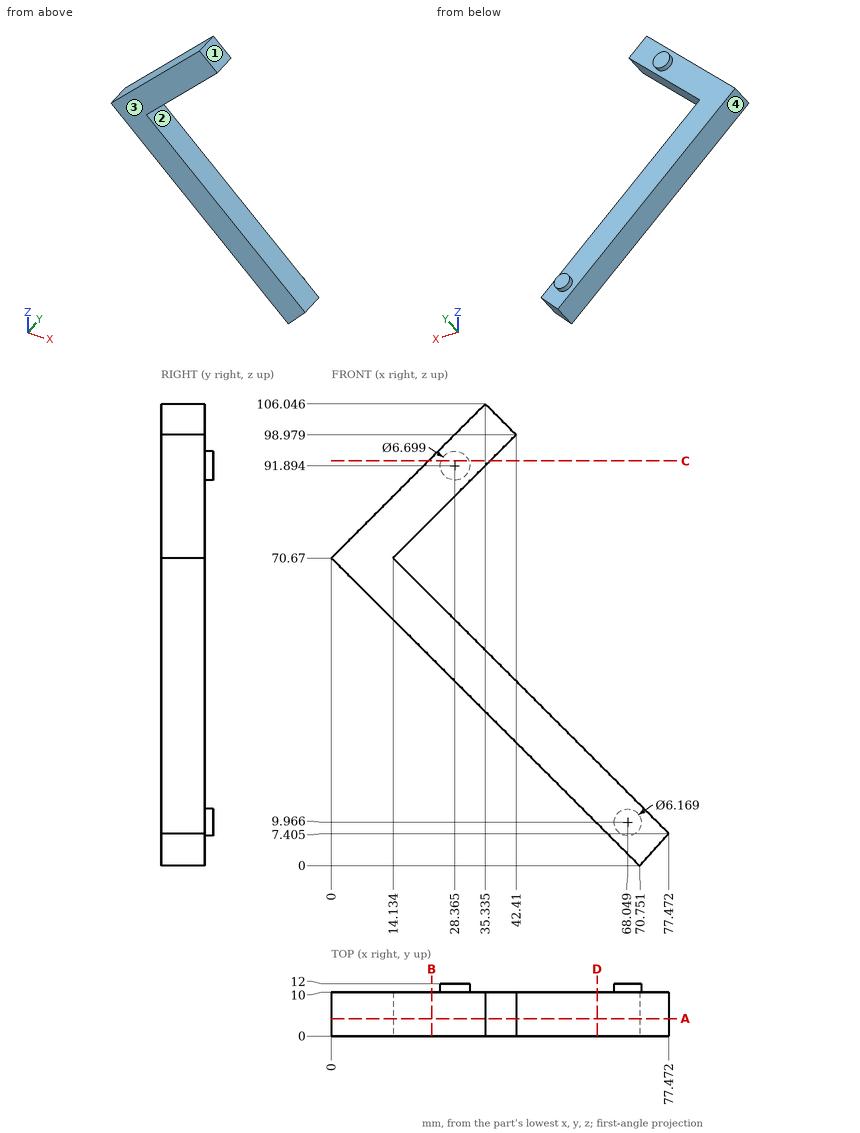
Source: three-view drawing plus pictorial views. Frame: mm from the lowest corner of the part. Coordinates: 2 decimals unless noted, no trailing zeros. Loops run counter-clockwise (first coordinate to the right, second up) from the corner with the lowest first, then second, coordinate; pieces in that order, holes last. Notation, with made-up numbers: (75.25, -22.5) - (108.25, -22.5) arc R28 ccw to (108.25, -1.5) - close; hole circle Ø3 at (-20, -22.75). An arc over 180 degrees is marked (long way). Answer in a Markdown table with one row per item. Add a question column.
Item 1: Section query C-C on z = 93. Return the cut outline in (x, y) (1 decimal), then the cut area to 3 significant figures.
Item 2: Line query: line 1 along Z through (x, y) = (37.5, 6.75) (1 decimal); line 2 along Z through (x, y) = (31.5, 6) (1 decimal); line 3 along Y through (x, z) = (36, 38.5). Output: solid intervals per line, ascending. Write a range as [from, to].
Item 3: Section query A-A on y = 4. Return the cut outline in (x, z) (1 decimal).
Item 4: Section query B-B on x = 23. Return the cut outline in (y, z) (1 decimal).
Item 5: Contact query for flat-ended pins moving along their axis: P1, Ø4, axis at x = 58, y = 5.5, coming from the -Z side; P2, Ø1, axis at x = 51.5, y = 3, coming from the +Z side (1 decimal); P3, Ø6, axis at x = 51, y = 8.5, coming from the +Z side (1 decimal). Output: stop coordinate, or through.
Item 6: Section query D-D on x = 61. Return the cut outline in (y, z).
Item 7: Mould query, pull axis Z, two halves, no side actions, for the marked faces 1, 2, 3 and 4. Classes: released by +Z, released by -Z, zero draft, split by the parting line, or undercut.
Recorded:
| question | item | result |
|---|---|---|
| 1 | outline | (22.3, 0) - (36.4, 0) - (36.4, 10) - (31.5, 10) - (31.5, 12) - (25.2, 12) - (25.2, 10) - (22.3, 10) - close |
| 1 | area | 154 mm^2 |
| 2 | line 1 | [33.2, 47.3], [94.1, 103.9] |
| 2 | line 2 | [39.2, 53.3], [88.1, 102.2] |
| 2 | line 3 | [0, 10] |
| 3 | outline | (0, 70.7) - (70.8, 0) - (77.5, 7.4) - (14.1, 70.7) - (42.4, 99) - (35.3, 106) - close |
| 4 | outline | (0, 47.7) - (10, 47.7) - (10, 61.8) - (0, 61.8) - close; (0, 79.5) - (10, 79.5) - (10, 93.7) - (0, 93.7) - close |
| 5 | P1 | z = 10.74 |
| 5 | P2 | z = 33.8 |
| 5 | P3 | z = 36.8 |
| 6 | outline | (0, 9.74) - (10, 9.74) - (10, 23.86) - (0, 23.86) - close |
| 7 | face 1 | released by +Z |
| 7 | face 2 | undercut |
| 7 | face 3 | zero draft |
| 7 | face 4 | released by -Z |
